```python
from build123d import *

# Parameters (mm, degrees)
F1_DEPTH = 45
F3_R     = 2.5
F4_DEPTH = 6


with BuildPart() as f1:
    # F0 (on Top) → F1 (new body)
    with BuildSketch(Plane.XY):
        with BuildLine():
            ThreePointArc((-4.242641, 4.242641), (5.977132, 0.523351), (-3.440774, -4.915392))
            Line((-3.440774, -4.915392), (-5.734623, -8.192319))
            ThreePointArc((-5.734623, -8.192319), (4.618104, -8.869787), (10, 0))
            Line((10, 0), (10, 39))
            ThreePointArc((10, 39), (9.707107, 39.707107), (9, 40))
            Line((9, 40), (5, 40))
            ThreePointArc((5, 40), (4.292893, 39.707107), (4, 39))
            Line((4, 39), (4, 19.078784))
            ThreePointArc((4, 19.078784), (2.062258, 13.162704), (-3, 9.539392))
            ThreePointArc((-3, 9.539392), (-5.184569, 8.551037), (-7.071068, 7.071068))
            Line((-7.071068, 7.071068), (-4.242641, 4.242641))
        make_face()
    extrude(amount=F1_DEPTH)

    # F3 (on face) → F4 (cut)
    with BuildSketch(Plane.YZ.offset(10)):
        with Locations((25.139775, 32.5)):
            Circle(F3_R)
        with Locations((25.139775, 12.5)):
            Circle(F3_R)
    extrude(amount=-F4_DEPTH, mode=Mode.SUBTRACT)


solid = f1.part
```
Design review of the part built by this model. Coordinates are the model's own, in mm. A direction names the side the tool comes from. Give positions to 0.01 mm unless a question says otherwise; leave off trailing zeros. Loops run counter-clockwise (first coordinate to the right, second up) from the corner with the lowest first, then second, coordinate; pieces in that order, holes last. Notation, with made-up numbers: (26.5, -35.5) -> (62.5, -35.5) arc R17 cw to (62.5, -2.5) -> close; hole circle Ø7 at (-35, 46). An arc over 180 degrees is marked (long way). One line per item, written item: value.
Q1. We need section D-D on x = 0. Give the boundary of the cut face in (y, z).
Numbers:
outline: (-10, 0) -> (-6, 0) -> (-6, 45) -> (-10, 45) -> close; (6, 0) -> (11.08, 0) -> (11.08, 45) -> (6, 45) -> close
Q2. For L1, parallel to Z at x = 7.75, y = 25; L2, parallel to X at y = 0, z = 11; L3, parallel to Y at x = -1, z = 36, list the stretches that pass through material, from the lowest coordinate up.
Numbers:
L1: z = 0 to 10, 15 to 30, 35 to 45
L2: x = 6 to 10
L3: y = -9.95 to -5.92, 5.92 to 10.42
Q3. Draft analysis for pull direction X (two halves, no side actions). For faces 4 (the cylindrical face through (7.04, 26.29, 10.28)), 5 (the cylindrical face through (5.957, 0.713, 22.185)), 6 (the flat face through (10, 19, 22)), state which applies: pulls with the +X half, pulls with the -X half, needs draft (parallel to the pull), parting line crosses it, or undercut.
Numbers:
face 4: needs draft
face 5: undercut
face 6: pulls with the +X half
Q4. We need section B-B on x = -5. Give the boundary of the cut face in (y, z).
Numbers:
outline: (-8.66, 0) -> (-7.14, 0) -> (-7.14, 45) -> (-8.66, 45) -> close; (5, 0) -> (8.66, 0) -> (8.66, 45) -> (5, 45) -> close
Q5. We need section C-C on z = 5.5. Give the boundary of the cut face in (x, y), and give its area (3 significant figures).
Numbers:
outline: (-7.07, 7.07) -> (-4.24, 4.24) arc R6 cw (long way) to (-3.44, -4.92) -> (-5.73, -8.19) arc R10 ccw to (10, 0) -> (10, 39) arc R1 ccw to (9, 40) -> (5, 40) arc R1 ccw to (4, 39) -> (4, 19.08) arc R10 cw to (-3, 9.54) arc R10 ccw to start
area: 361 mm^2
Q6. We need section A-A on z = 32.5. Give the boundary of the cut face in (x, y), and give its area (3 significant figures).
Numbers:
outline: (-7.07, 7.07) -> (-4.24, 4.24) arc R6 cw (long way) to (-3.44, -4.92) -> (-5.73, -8.19) arc R10 ccw to (10, 0) -> (10, 22.64) -> (4, 22.64) -> (4, 19.08) arc R10 cw to (-3, 9.54) arc R10 ccw to start; (4, 27.64) -> (10, 27.64) -> (10, 39) arc R1 ccw to (9, 40) -> (5, 40) arc R1 ccw to (4, 39) -> close
area: 331 mm^2
Q7. Machinability: for faces 1 (the flat face through (-6, 6, 22)), 2 (the flat face through (4, 29, 22)), 3 (the flat face through (5, 15, 0)), which of the approach directions +Z, -Z, +X, -X, +Y, -Y give a long, thin tool a straight path to every point of the face, cutting with its end or side? Answer none if there is none.
Numbers:
face 1: +Z, -Z, -X
face 2: +Z, -Z, -X, +Y
face 3: -Z, +X, -X, +Y, -Y
Q8. For pin 1 Ø16 at (y, z) = (25.5, 11.5) entering from -X; pin 2 Ø4 at (y, z) = (27, 8.5) entering from -X; pin 3 Ø3 at (y, z) = (-2, 32.5) entering from +X; pin 4 Ø4 at (y, z) = (25.14, 32.5) entering from -X, all flat-tipped, find the tip position at first contact; note any pin that passes through.
Numbers:
pin 1: stops at x = 3.87
pin 2: stops at x = 4
pin 3: stops at x = 9.99
pin 4: passes through
